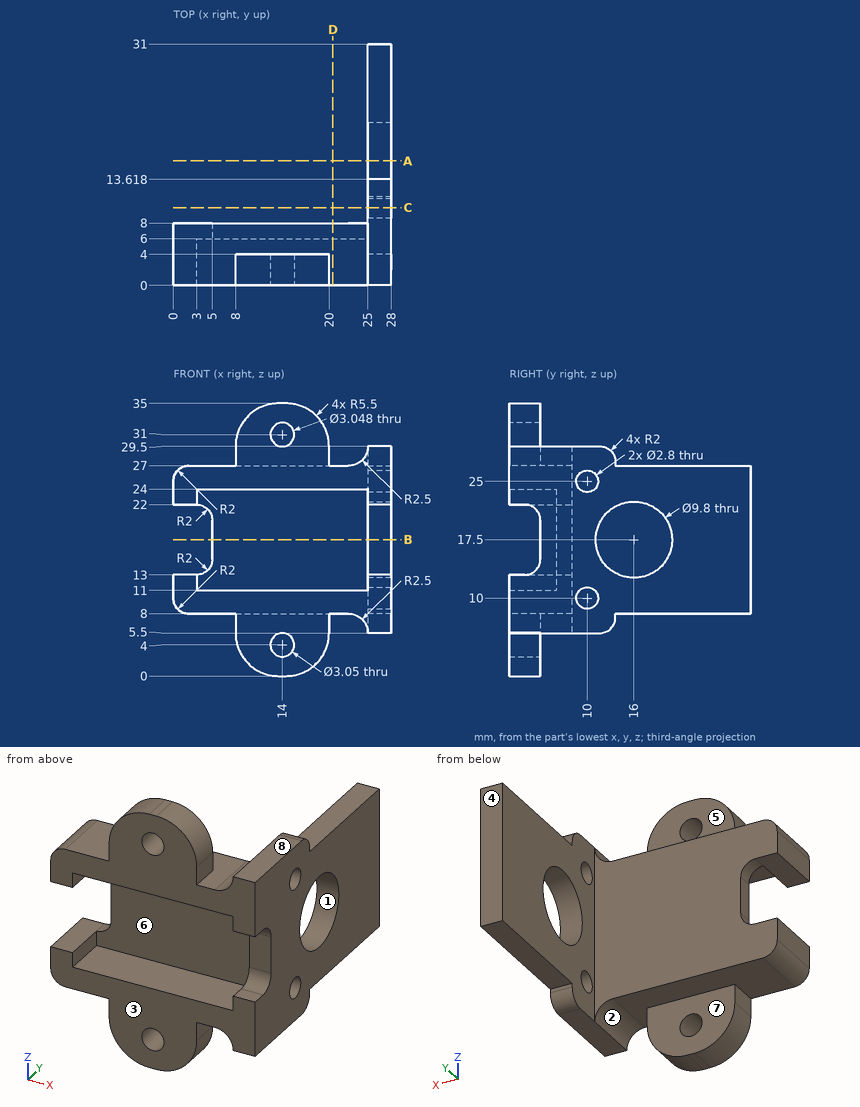
Answer from the drawing. Dimensions are ordinates in mm from the lowest x, y and z of the part. A direction names the side the tool comes from. Coordinates: 2 decimals unless noted, no trailing zeros. Write each loop counter-clockwise with the first axis right and the second up, starting at its lowest first coordinate (ties: lowest second). Pieces come first, ordered by that corner, then holes. Notation, with made-up numbers: (41, 21) - (61, 21) arc R28 ccw to (61, 53) - close; hole circle Ø6 at (47.25, -2.5). An arc over 180 degrees is marked (long way). Return JSON: item names as keys, results as strings. Group by question number.
Q1. Flat-ended cylindrical pins translate along their axes: pin 1 Ø2 at (y, z) = (7.5, 16.5) entering from -X; pin 2 Ø4 at (x, z) = (14.5, 32) entering from +Y; pin 3 Ø8 at (x, y) = (24.5, 27.5) entering from +Z. Find the tip coordinate at first contact, or state that the pin passes through.
Q2. The part is cut by section B-B on z = 17.5. Write down the section's boundary in (x, y), and give its area (3 significant figures).
Q3. Find the intervals of material crossed by line 1 along Y through (x, z) = (26.25, 10); line 2 along X through (y, z) = (11, 27.5); line 3 along Y through (x, z) = (10.5, 6.5), in increasing order. Write a range as [from, to].
Q4. The part is cut by section C-C on y = 10. Write down the section's boundary in (x, z), and give its area (3 significant figures).
Q5. For a pull along Y with two mould halves and no side action, classify the marked faces 1, 2, 3 and 4 as +Y half, -Y half, draft (parallel to the pull), parting line (faces both ways), or undercut.
Q6. The part is cut by section D-D on x = 20.5. Write down the section's boundary in (y, z).
Q7. The part is cut by section A-A on y = 16. Write down the section's boundary in (x, z).
Q8. Which of the six approach directions +Z, -Z, +X, -X, +Y, -Y give full straight-line access (tool end or side, diameter ignored) to the marked faces 5, 6, 7 and 8?
Evaluation:
{
 "1": {"pin 1": "stops at x = 5", "pin 2": "stops at y = 4", "pin 3": "stops at z = 27"},
 "2": {"outline": "(5, 6) - (25, 6) - (25, 4) - (28, 4) - (28, 11.1) - (25, 11.1) - (25, 8) - (5, 8) - close; (25, 20.9) - (28, 20.9) - (28, 31) - (25, 31) - close", "area": "91.6 mm2"},
 "3": {"line 1": "y = [0, 8.6], [11.4, 31]", "line 2": "x = [25, 28]", "line 3": "y = [0, 4]"},
 "4": {"outline": "(25, 5.5) - (28, 5.5) - (28, 8.6) - (25, 8.6) - close; (25, 11.4) - (28, 11.4) - (28, 23.6) - (25, 23.6) - close; (25, 26.4) - (28, 26.4) - (28, 29.5) - (25, 29.5) - close", "area": "55.2 mm2"},
 "5": {"face 1": "undercut", "face 2": "draft", "face 3": "-Y half", "face 4": "+Y half"},
 "6": {"outline": "(0, 8) - (8, 8) - (8, 27) - (0, 27) - (0, 24) - (6, 24) - (6, 11) - (0, 11) - close"},
 "7": {"outline": "(25, 8) - (28, 8) - (28, 12.6) - (25, 12.6) - close; (25, 22.4) - (28, 22.4) - (28, 27) - (25, 27) - close"},
 "8": {"face 5": "+Z, -X, +Y", "face 6": "-Y", "face 7": "-Z, -X, +Y", "face 8": "+Z, +X, +Y, -Y"}
}
